from build123d import *

# Parameters (mm, degrees)
CROQUIS1_W              = 9
CROQUIS1_H              = 20.3
SALIENTE_EXTRUIR1_DEPTH = 9
CROQUIS2_W              = 7
CROQUIS2_H              = 18.3
CORTAR_EXTRUIR1_DEPTH   = 6.5
CROQUIS3_W              = 18.3
CROQUIS3_H              = 9
CORTAR_EXTRUIR2_DEPTH   = 0.2
CROQUIS4_W              = 4.2
CROQUIS4_H              = 7.7
CORTAR_EXTRUIR3_DEPTH   = 1
CROQUIS5_W              = 0.5
CROQUIS5_H              = 0.5
SALIENTE_EXTRUIR2_DEPTH = 10
CROQUIS6_W              = 0.5
CROQUIS6_H              = 0.5
SALIENTE_EXTRUIR3_DEPTH = 2.5


with BuildPart() as part:
    # Croquis1 → Saliente-Extruir1 (new body)
    with BuildSketch(Plane(origin=(0, 0, 0), x_dir=(1, 0, 0), z_dir=(0, 1, 0))):
        with Locations((4.5, 10.15)):
            Rectangle(CROQUIS1_W, CROQUIS1_H)
    extrude(amount=SALIENTE_EXTRUIR1_DEPTH)

    # Croquis2 → Cortar-Extruir1 (cut)
    with BuildSketch(Plane(origin=(0, 9, 0), x_dir=(1, 0, 0), z_dir=(0, 1, 0))):
        with Locations((4.5, 10.15)):
            Rectangle(CROQUIS2_W, CROQUIS2_H)
    extrude(amount=-CORTAR_EXTRUIR1_DEPTH, mode=Mode.SUBTRACT)

    # Croquis3 → Cortar-Extruir2 (cut)
    with BuildSketch(Plane(origin=(9, 0, 0), x_dir=(0, 0, -1), z_dir=(1, 0, 0))):
        with Locations((10.15, 4.5)):
            Rectangle(CROQUIS3_W, CROQUIS3_H)
    extrude(amount=-CORTAR_EXTRUIR2_DEPTH, mode=Mode.SUBTRACT)

    # Croquis4 → Cortar-Extruir3 (cut)
    with BuildSketch(Plane.ZY):
        with Locations((-10.15, 5.15)):
            Rectangle(CROQUIS4_W, CROQUIS4_H)
    extrude(amount=-CORTAR_EXTRUIR3_DEPTH, mode=Mode.SUBTRACT)

    # Croquis5 → Saliente-Extruir2 (add)
    with BuildSketch(Plane(origin=(0, 9, 0), x_dir=(1, 0, 0), z_dir=(0, 1, 0))):
        with Locations((5.8, 15.15)):
            Rectangle(CROQUIS5_W, CROQUIS5_H)
        with Locations((3.2, 15.15)):
            Rectangle(CROQUIS5_W, CROQUIS5_H)
        with Locations((5.8, 12.65)):
            Rectangle(CROQUIS5_W, CROQUIS5_H)
        with Locations((5.8, 10.15)):
            Rectangle(CROQUIS5_W, CROQUIS5_H)
        with Locations((5.8, 7.65)):
            Rectangle(CROQUIS5_W, CROQUIS5_H)
        with Locations((5.8, 5.15)):
            Rectangle(CROQUIS5_W, CROQUIS5_H)
        with Locations((3.2, 12.65)):
            Rectangle(CROQUIS5_W, CROQUIS5_H)
        with Locations((3.2, 10.15)):
            Rectangle(CROQUIS5_W, CROQUIS5_H)
        with Locations((3.2, 7.65)):
            Rectangle(CROQUIS5_W, CROQUIS5_H)
        with Locations((3.2, 5.15)):
            Rectangle(CROQUIS5_W, CROQUIS5_H)
    extrude(amount=-SALIENTE_EXTRUIR2_DEPTH)

    # Croquis6 → Saliente-Extruir3 (add)
    with BuildSketch(Plane.ZY.offset(-2.95)):
        with Locations((-5.15, -0.75)):
            Rectangle(CROQUIS6_W, CROQUIS6_H)
        with Locations((-7.65, -0.75)):
            Rectangle(CROQUIS6_W, CROQUIS6_H)
        with Locations((-10.15, -0.75)):
            Rectangle(CROQUIS6_W, CROQUIS6_H)
        with Locations((-12.65, -0.75)):
            Rectangle(CROQUIS6_W, CROQUIS6_H)
        with Locations((-15.15, -0.75)):
            Rectangle(CROQUIS6_W, CROQUIS6_H)
    saliente_extruir3 = extrude(amount=SALIENTE_EXTRUIR3_DEPTH)

    # Simetría1: Saliente-Extruir3 across plane
    add(saliente_extruir3.mirror(Plane(origin=(4.5, 0, 0), x_dir=(0, 0, 1), z_dir=(1, 0, 0))))


solid = part.part
Could you check a few things on this model? Use its own coordinates, in mm. A direction names the side the tool comes from. Round coordinates to 2 decimals unless told otherwise and drop trailing zeros. Write each loop counter-clockwise with the first axis right and the second up, starting at its lowest first coordinate (ties: lowest second). Pieces come first, ordered by that corner, then holes. Notation, with made-up numbers: (88, 32) - (99, 32) arc R28 ccw to (99, 58) - close; hole circle Ø4 at (69.25, 77.25). An arc over 180 degrees is marked (long way). Put each result on its own line as item: value. Start each with the question number.
(1) I want a section at B-B, the plane z = -18.5. Please give me the cut outline in (x, y).
(2) I want a section at A-A, the plane x = 6.75. Please give me the cut outline in (y, z).
(3) I need wall thicknesses on probe 1 along X at (y, z) = (5, -7.5); probe 2 along X at (y, z) = (6.5, -10); probe 3 along Y at (x, z) = (0.5, -5). Which ranges of each line are inside material? Lowest first, please.
(4) For faces 1 (the flat face through (0.5, 1.3, -10.2)), 2 (the flat face through (4, 6, -1)), 3 (the flat face through (1.9, -0.7, -15.4)), 4 (the flat face through (8.15, 9, -10.95)), 5 (the flat face through (6.7, -0.7, -5.4)), which set-ups out of +Z, -Z, +X, -X, +Y, -Y let a thin tool reach every point of the face, with its end or its side?
(5) Will these pins go through, and if not, where does the flat tip stop? pin 1 (2 mm diameter, centred on x = 5.5, z = -3, fed in from -Y); pin 2 (0.6 mm diameter, centred on y = 5.5, z = -10, fed in from +X); pin 3 (0.8 mm diameter, centred on x = 7.5, y = -0.5, fed in from -Z).
(6) Thinking about a two-plate mould opening in X: for faces 6 (the flat face through (6.7, -0.7, -7.4)), 7 (the flat face through (4, 6, -19.3)), 8 (the flat face through (9, 4, -20)), which applies, released by +X, released by -X, zero draft, split by the parting line, or undercut?
(7) I want a section at D-D, the plane y = 3.5. Give the number of separate pieces and of enclosed holes in the cut face, plus the area to 3 significant figures.
(8) I want a section at C-C, the plane x = 5.25. Please give me the cut outline in (y, z), plus the area to 4 significant figures.
Here are the results:
1. outline: (0, 0) - (8.8, 0) - (8.8, 9) - (8, 9) - (8, 2.5) - (1, 2.5) - (1, 9) - (0, 9) - close
2. outline: (-1, -15.4) - (-0.5, -15.4) - (-0.5, -14.9) - (-1, -14.9) - close; (-1, -12.9) - (-0.5, -12.9) - (-0.5, -12.4) - (-1, -12.4) - close; (-1, -10.4) - (-0.5, -10.4) - (-0.5, -9.9) - (-1, -9.9) - close; (-1, -7.9) - (-0.5, -7.9) - (-0.5, -7.4) - (-1, -7.4) - close; (-1, -5.4) - (-0.5, -5.4) - (-0.5, -4.9) - (-1, -4.9) - close; (0, -20.3) - (9, -20.3) - (9, -19.3) - (2.5, -19.3) - (2.5, -1) - (9, -1) - (9, 0) - (0, 0) - close
3. probe 1: x = 0 to 1, 2.95 to 3.45, 5.55 to 6.05, 8 to 8.8
3. probe 2: x = 2.95 to 3.45, 5.55 to 6.05, 8 to 8.8
3. probe 3: y = -1 to -0.5, 0 to 9
4. face 1: -X, +Y
4. face 2: +Y
4. face 3: -Z, +X, -X, -Y
4. face 4: +Z, -Z, +X, -X, +Y
4. face 5: +X, -X, -Y
5. pin 1: stops at y = 0
5. pin 2: stops at x = 8.8
5. pin 3: stops at z = -15.4
6. face 6: zero draft
6. face 7: undercut
6. face 8: released by +X
7. separate pieces: 11
7. enclosed holes: 0
7. area: 49.2 mm^2
8. outline: (0, -20.3) - (9, -20.3) - (9, -19.3) - (2.5, -19.3) - (2.5, -1) - (9, -1) - (9, 0) - (0, 0) - close
8. area: 63.75 mm^2
